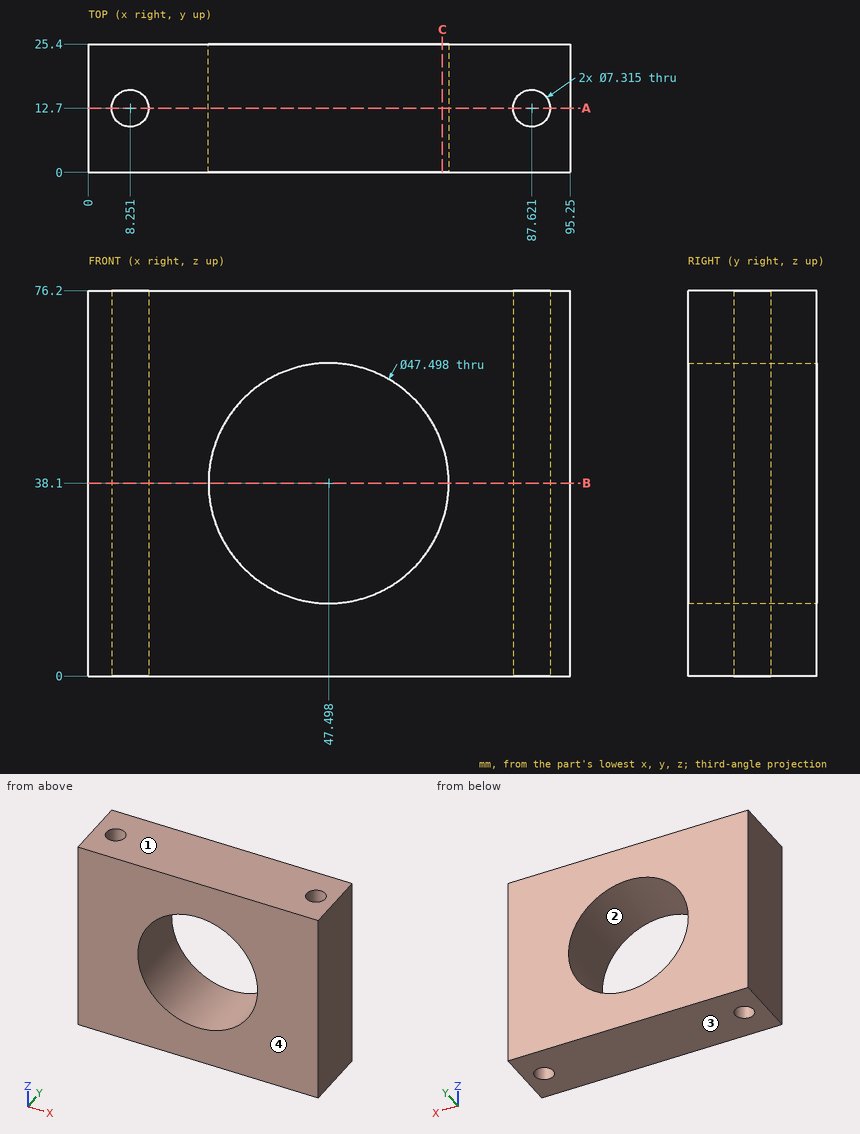
Geometry check sheet. Reference: drawing and pictorial views, mm from the part's lowest x, y, z. Round coordinates to 2 decimals unless told otherwise and drop trailing zeros. Loops run counter-clockwise (first coordinate to the right, second up) from the corner with the lowest first, then second, coordinate; pieces in that order, holes last. Notation, with made-up numbers: M 8,78 L 66,78 A6 ccw 66,82 Z; hole C -23,-12 d9. An arc over 180 degrees is marked long. One line per item, written item: value.
(1) Release check for a two-part mould opening along Z. For the marked faces 1, 2, 3 and 4 record: +Z half, -Z half, draft (parallel to the pull), parting line (faces both ways), or undercut.
Computed values:
face 1: +Z half
face 2: undercut
face 3: -Z half
face 4: draft
(2) Thickness scan on line 1 (Z direction, x = 47, y = 5); line 2 (X direction, y = 11, z = 30.5); line 3 (Z direction, x = 33.5, y = 21) (1 decimal). Record the ranges inside material, lowest first.
Computed values:
line 1: z = 0 to 14.36, 61.84 to 76.2
line 2: x = 0 to 5.01, 11.49 to 25, 70 to 84.38, 90.86 to 95.25
line 3: z = 0 to 18.9, 57.3 to 76.2
(3) Sectioned sample at C-C, the plane x = 70. Record the cut outline in (y, z) (1 decimal), then the cut area to 3 significant figures.
Computed values:
outline: M 0,0 L 25.4,0 L 25.4,30.5 L 0,30.5 Z; M 0,45.7 L 25.4,45.7 L 25.4,76.2 L 0,76.2 Z
area: 1,550 mm^2
(4) Sectioned sample at A-A, the plane y = 12.7. Record the cut outline in (x, z), then the cut area to 3 significant figures.
Computed values:
outline: M 0,0 L 4.59,0 L 4.59,76.2 L 0,76.2 Z; M 11.91,0 L 83.96,0 L 83.96,76.2 L 11.91,76.2 Z; M 91.28,0 L 95.25,0 L 95.25,76.2 L 91.28,76.2 Z; hole C 47.5,38.1 d47.5
area: 4,370 mm^2
(5) Sectioned sample at B-B, the plane z = 38.1. Count the separate pieces of the cut face and the enclosed holes in it, then the cut area to 3 significant figures.
Computed values:
separate pieces: 2
enclosed holes: 2
area: 1,130 mm^2
